from build123d import *

# Parameters (mm, degrees)
CROQUIS1_W              = 42
CROQUIS1_H              = 85
CROQUIS1_R              = 2.05
CROQUIS1_R_2            = 2.55
SALIENTE_EXTRUIR1_DEPTH = 4
CROQUIS5_R              = 11.5
CROQUIS5_R_2            = 1.575
CORTAR_EXTRUIR2_DEPTH   = 5
CROQUIS7_W              = 42
CROQUIS7_H              = 7.7
SALIENTE_EXTRUIR2_DEPTH = 4
CHAFL_N1_SIZE           = 4.1


with BuildPart() as part:
    # Croquis1 → Saliente-Extruir1 (new body)
    with BuildSketch(Plane.XY):
        with Locations((21, 42.5)):
            Rectangle(CROQUIS1_W, CROQUIS1_H)
        with Locations((11, 76.8)):
            Circle(CROQUIS1_R, mode=Mode.SUBTRACT)
        with Locations((31, 76.8)):
            Circle(CROQUIS1_R, mode=Mode.SUBTRACT)
        with Locations((31, 56.8)):
            Circle(CROQUIS1_R, mode=Mode.SUBTRACT)
        with Locations((11, 56.8)):
            Circle(CROQUIS1_R, mode=Mode.SUBTRACT)
        with Locations((21, 21.08)):
            Circle(CROQUIS1_R_2, mode=Mode.SUBTRACT)
    extrude(amount=SALIENTE_EXTRUIR1_DEPTH)

    # Croquis5 → Cortar-Extruir2 (cut, through all)
    with BuildSketch(Plane.XY.offset(4)):
        with Locations((21, 21.08)):
            Circle(CROQUIS5_R)
        with Locations((5.5, 36.58)):
            Circle(CROQUIS5_R_2)
        with Locations((36.5, 36.58)):
            Circle(CROQUIS5_R_2)
        with Locations((36.5, 5.58)):
            Circle(CROQUIS5_R_2)
        with Locations((5.5, 5.58)):
            Circle(CROQUIS5_R_2)
    extrude(amount=-CORTAR_EXTRUIR2_DEPTH, mode=Mode.SUBTRACT)

    # Croquis7 → Saliente-Extruir2 (add, through all)
    with BuildSketch(Plane.XY.offset(4)):
        with Locations((21, -3.85)):
            Rectangle(CROQUIS7_W, CROQUIS7_H)
    extrude(amount=-SALIENTE_EXTRUIR2_DEPTH)

    # Chaflán1
    chafl_n1_edges = [part.edges().sort_by_distance(p)[0] for p in [
        (0, -7.7, 2),
        (42, -7.7, 2),
    ]]
    chamfer(chafl_n1_edges, length=CHAFL_N1_SIZE)


solid = part.part
Input: part model. Units: mm. Frame: model coordinates. Give positions to 0.01 mm unless a question says otherwise; leave off trailing zeros. Write each loop counter-clockwise with the first axis right and the second up, starting at its lowest first coordinate (ties: lowest second). Pieces come first, ordered by that corner, then holes.
Q1. Pull-direction query (Y, two-part tool) for faces 1 (the face through (31.623, 16.675, 2.028)), 2 (the face through (39.9, -5.7, 2)), 3 (the face through (42, 40, 2)); classes: pulls with the +Y half, pulls with the -Y half, needs draft (parallel to the pull), parting line crosses it, or undercut.
Q2. Section C-C, the plane x = 36.5. Output: boundary loops of the cut face in (y, z) (3 decimals).
Q3. Section D-D, the plane z = 1.9. State how many separate pieces and enclosed holes the cut face has, plus the area to 3 significant figures.
Q4. Section A-A, the plane y = 5.58. Output: boundary loops of the cut face in (x, z) (3 decimals), plus the area to 3 significant figures.
Q5. Material intervals for probe 1 along Y at (x, z) = (5.5, 1.95) (3 decimals); probe 2 along Y at (x, z) = (21, 2.75); probe 3 along Y at (x, z) = (11, 2.4), sorted ascending.
Q6. Section B-B, the plane x = 21. Output: boundary loops of the cut face in (y, z), plus the area to 3 significant figures.
Q7. First-contact query: P1, Ø3.5, axis at x = 11, y = 76.8, coming from the -Z side. Flat tip, straight axial feed; report the tip coordinate or a pass-through.
Filled in:
1. face 1: undercut
1. face 2: pulls with the -Y half
1. face 3: needs draft
2. outline: (-7.7, 0) - (4.005, 0) - (4.005, 4) - (-7.7, 4) - close; (7.155, 0) - (35.005, 0) - (35.005, 4) - (7.155, 4) - close; (38.155, 0) - (85, 0) - (85, 4) - (38.155, 4) - close
3. separate pieces: 1
3. enclosed holes: 9
3. area: 3,380 mm2
4. outline: (0, 0) - (3.925, 0) - (3.925, 4) - (0, 4) - close; (7.075, 0) - (34.925, 0) - (34.925, 4) - (7.075, 4) - close; (38.075, 0) - (42, 0) - (42, 4) - (38.075, 4) - close
4. area: 143 mm2
5. probe 1: y = -7.7 to 4.005, 7.155 to 35.005, 38.155 to 85
5. probe 2: y = -7.7 to 9.58, 32.58 to 85
5. probe 3: y = -7.7 to 15.4, 26.76 to 54.75, 58.85 to 74.75, 78.85 to 85
6. outline: (-7.7, 0) - (9.58, 0) - (9.58, 4) - (-7.7, 4) - close; (32.58, 0) - (85, 0) - (85, 4) - (32.58, 4) - close
6. area: 279 mm2
7. P1: passes through
